Read the model definition and answer for the solid it produces. Units are mm, in the model's axes. Give positions to 0.01 mm unless a question says otherwise; leave off trailing zeros. Order: outer loops, then holes, each group sorted by start corner. A loop starts at its lowest first (then second) coordinate and runs counter-clockwise, first axis right, second up. Notation, with made-up numbers: (43.5, -32) - (50.5, -32) arc R20 ccw to (50.5, -26) - close; hole circle Ø11 at (69, 28.5). An arc over 180 degrees is marked (long way). Answer as CSV lines item,"result". Start each with the question number.
from build123d import *

# Parameters (mm, degrees)
ESQUISSE1_W        = 2.8
ESQUISSE1_H        = 4.8
BOSS_EXTRU_1_DEPTH = 1


with BuildPart() as part:
    # Esquisse1 → Boss.-Extru.1 (new body)
    with BuildSketch(Plane(origin=(0, 0, 0), x_dir=(1, 0, 0), z_dir=(0, 1, 0))):
        Rectangle(ESQUISSE1_W, ESQUISSE1_H)
    extrude(amount=BOSS_EXTRU_1_DEPTH)

    # Esquisse2 → Révolution1 (revolve)
    with BuildSketch(Plane(origin=(0, 0, 0), x_dir=(0, 0, -1), z_dir=(1, 0, 0))):
        Polygon((0, 0), (0, 100), (22.169466264, 100), align=None)
    revolve(axis=Axis((0, 0, 0), (0, 1, 0)))


solid = part.part
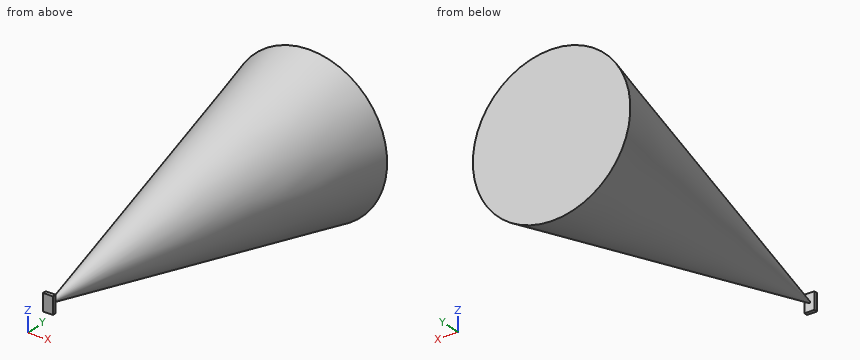
(1) Section B-B, the plane y = 19 is taken. Write down the section's boundary in (x, z), and give its area (3 significant figures).
(2) Section A-A, the plane y = 63.5 is taken. Write down the section's boundary in (x, z).
(3) Flat-ended cylindrical pins translate along their axes: pin 1 Ø6 at (y, z) = (51, -17) entering from +X; pin 2 Ø0.8 at (x, y) = (0.5, 0.5) entering from -Z; pin 3 Ø4 at (x, y) = (9.5, 70.5) entering from +Z; pin 4 Ø0.5 at (x, y) = (0.5, 0.5) entering from +Z. Find the tip coordinate at first contact, or state that the pin passes through.
(4) Straight lines are drawn through the part: line 1 (Z direction, x = 0, y = 95); line 2 (X direction, y = 89, z = -0.5); line 3 (X direction, y = 13, z = -2.5). For each, find the intervals that lie inside material, in ascending order. Write a range as [from, to].
Checks:
1,outline,"circle Ø8.42 at (0, 0)"
1,area,"55.7 mm²"
2,outline,"circle Ø28.16 at (0, 0)"
3,pin 1,"passes through"
3,pin 2,"stops at z = -2.4"
3,pin 3,"stops at z = 13.82"
3,pin 4,"stops at z = 2.4"
4,line 1,"z = [-21.06, 21.06]"
4,line 2,"x = [-19.72, 19.72]"
4,line 3,"x = [-1.43, 1.43]"
